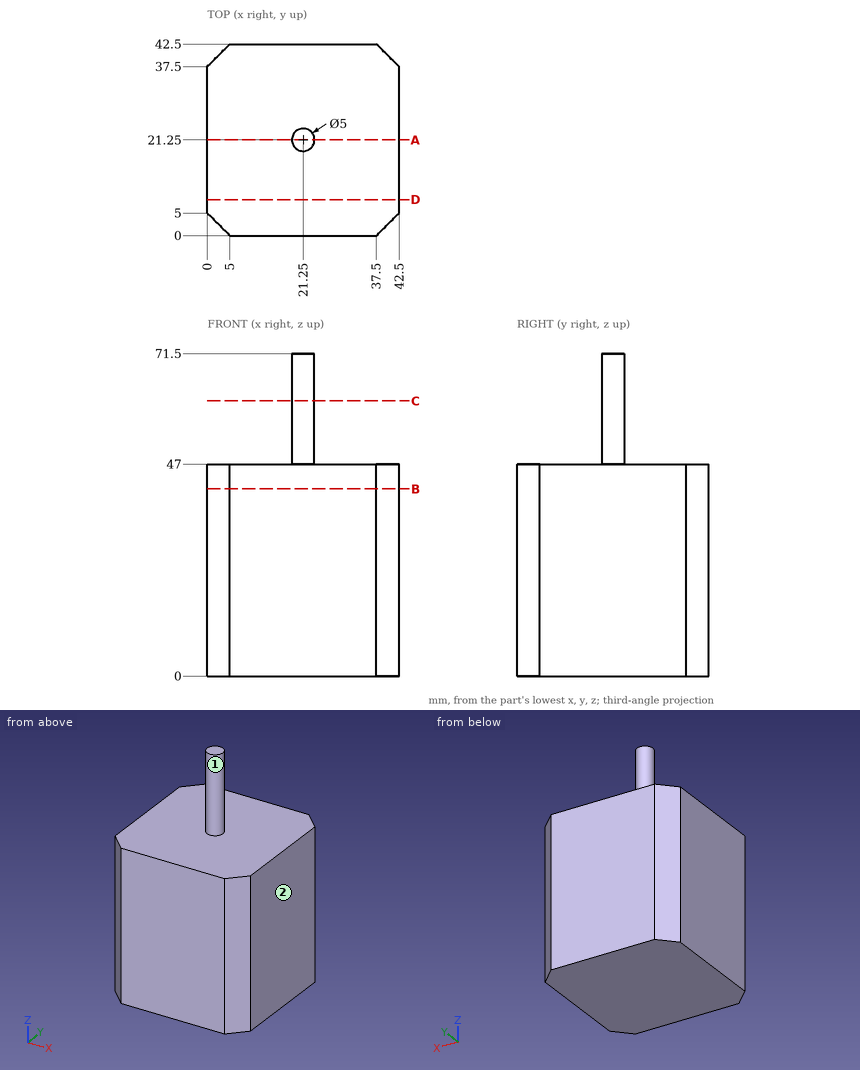
Design review of the part shown in the three views and the two pictorial views. Dimensions are in mm from the part's minimum x, y and z. A direction names the side the tool comes from. Round coordinates to 2 decimals unless told otherwise and drop trailing zeros. Write each loop counter-clockwise with the first axis right and the second up, starting at its lowest first coordinate (ties: lowest second). Pieces come first, ordered by that corner, then holes.
Item 1: Consider section D-D on y = 8. Give the boundary of the cut face in (x, z).
Item 2: For pin 1 Ø5 at (x, z) = (17.5, 31.5) entering from -Y; pin 2 Ø8 at (x, z) = (22.5, 53) entering from -Y, all flat-tipped, find the tip position at first contact; note any pin that passes through.
Item 3: Consider section C-C on z = 61. Give the boundary of the cut face in (x, y), and give its area (3 significant figures).
Item 4: Consider section B-B on z = 41.5. Give the boundary of the cut face in (x, y).
Item 5: Wall thickness on L1, parallel to Z at x = 6, y = 36.5; L2, parallel to X at y = 23, z = 59.5; L3, parallel to X at y = 3.5, z = 24: over which ranges is each line inside the solid? List them lowest first.
Item 6: For the marked faces 1 and 2, list the 3-axis set-ups (+Z, -Z, +X, -X, +Y, -Y) from which the entire face can be reached by the end or side of a thin tool; tool diameter is ignored.
Item 7: Consider section A-A on y = 21.25. Give the boundary of the cut face in (x, z).
Check values:
1. outline: (0, 0) - (42.5, 0) - (42.5, 47) - (0, 47) - close
2. pin 1: stops at y = 0
2. pin 2: stops at y = 18.75
3. outline: circle Ø5 at (21.25, 21.25)
3. area: 19.6 mm2
4. outline: (0, 5) - (5, 0) - (37.5, 0) - (42.5, 5) - (42.5, 37.5) - (37.5, 42.5) - (5, 42.5) - (0, 37.5) - close
5. L1: z = 0 to 47
5. L2: x = 19.46 to 23.04
5. L3: x = 1.5 to 41
6. face 1: +Z
6. face 2: +Z, -Z, +X, +Y, -Y
7. outline: (0, 0) - (42.5, 0) - (42.5, 47) - (23.75, 47) - (23.75, 71.5) - (18.75, 71.5) - (18.75, 47) - (0, 47) - close
